```python
from build123d import *

# Parameters (mm, degrees)
BOSS_EXTRUDE1_DEPTH        = 19.05
BOSS_EXTRUDE2_DEPTH        = 19.05
FILLET1_R                  = 3.175
FILLET2_R                  = 12.7
CUT_EXTRUDE1_DEPTH         = 965.552600368
CUT_EXTRUDE1_DEPTH_BACK    = 965.552600368
SKETCH47_R                 = 3.175
FILLET4_R                  = 6.35
F_0_25_DIAMETER_HOLE1_D    = 6.35
HOLE6_D                    = 3.175
HOLE6_DEPTH                = 38.1
HOLE6_CSINK_D              = 10.16
HOLE6_CSINK_ANGLE          = 82
HOLE6_TIP                  = 0.953866233
HOLE9_D                    = 3.175
HOLE9_DEPTH                = 57.15
HOLE9_CSINK_D              = 10.16
HOLE9_CSINK_ANGLE          = 82
HOLE9_TIP                  = 0.953866233
HOLE14_D                   = 3.175
HOLE14_DEPTH               = 31.75
HOLE14_CSINK_D             = 10.16
HOLE14_CSINK_ANGLE         = 82
HOLE14_TIP                 = 0.953866233
HOLE15_D                   = 3.175
HOLE15_DEPTH               = 31.75
HOLE15_CSINK_D             = 10.16
HOLE15_CSINK_ANGLE         = 82
HOLE15_TIP                 = 0.953866233
HOLE17_D                   = 3.175
HOLE17_DEPTH               = 31.75
HOLE17_CSINK_D             = 10.16
HOLE17_CSINK_ANGLE         = 82
HOLE17_TIP                 = 0.953866233
F_1_2_0_5_DIAMETER_HOLE3_D = 12.7


with BuildPart() as part:
    # Sketch1 → Boss-Extrude1 (new body)
    with BuildSketch(Plane.XY):
        Polygon((-247.274665566, 82.142339986), (-327.22102196, 55.917162383), (-560.337153612, 766.561933763), (-504.525442447, 784.870110692), (-417.251419261, 518.818903446), (-393.116774032, 526.735904121), align=None)
    extrude(amount=-BOSS_EXTRUDE1_DEPTH)

    # Sketch2 → Boss-Extrude2 (add, through all)
    with BuildSketch(Plane.XY):
        Polygon((-393.116774032, 526.735904121), (-336.901176267, 355.36500697), (-277.604402796, 374.816405204), (-281.415155825, 417.005352091), (-320.44916939, 493.083731154), (-290.280862854, 502.979981998), (-307.307307279, 554.884385267), align=None)
    extrude(amount=-BOSS_EXTRUDE2_DEPTH)

    # Fillet1
    fillet1_edges = [part.edges().sort_by_distance(p)[0] for p in [
        (-320.44916939, 493.083731154, -9.525),
    ]]
    fillet(fillet1_edges, radius=FILLET1_R)

    # Fillet2
    fillet2_edges = [part.edges().sort_by_distance(p)[0] for p in [
        (-336.901176267, 355.36500697, -9.525),
    ]]
    fillet(fillet2_edges, radius=FILLET2_R)

    # Sketch47 → Cut-Extrude1 (cut, two sides: drawn at the far end of the back side and taken through both)
    with BuildSketch(Plane(origin=(0, 0, -19.05), x_dir=(-1, 0, 0), z_dir=(0, 0, -1)).offset(-CUT_EXTRUDE1_DEPTH_BACK)):
        with Locations((417.251419261, 518.818903446)):
            Circle(SKETCH47_R)
    extrude(amount=CUT_EXTRUDE1_DEPTH + CUT_EXTRUDE1_DEPTH_BACK, mode=Mode.SUBTRACT)

    # Fillet4
    fillet4_edges = [part.edges().sort_by_distance(p)[0] for p in [
        (-418.241044345, 521.8357341, -9.525),
        (-414.234588607, 519.80852853, -9.525),
    ]]
    fillet(fillet4_edges, radius=FILLET4_R)

    # 0.25_ Diameter Hole1 (through all)
    with Locations(Plane.XY):
        with Locations((-563.45033927, 698.544682362), (-504.072834209, 517.534843147), (-343.557230523, 532.968767209), (-316.40575464, 541.875392969), (-305.317060721, 508.071973621), (-332.468536604, 499.165347862), (-384.427899865, 457.805801818), (-325.157897499, 477.248418201), (-305.715281117, 417.978415836), (-364.985283482, 398.535799453), (-323.698740376, 393.110483865), (-289.824308357, 404.222472403), (-287.772364418, 381.505347156), (-316.771364786, 371.99266929)):
            Hole(F_0_25_DIAMETER_HOLE1_D / 2)

    # Hole6
    with Locations(Plane(origin=(313.774034822, -375.700785937, -19.05), x_dir=(-0.9977564584489054, 0.06694811142592419, 0), z_dir=(0, 0, -1))):
        with Locations((615.24080496, 429.781381762), (710.914924699, 391.126528253), (904.68821492, 1078.38439498), (976.811864753, 1049.244548945), (835.937309391, 717.51890547), (711.83598555, 767.659094962)):
            CounterSinkHole(HOLE6_D / 2, HOLE6_CSINK_D / 2, depth=HOLE6_DEPTH, counter_sink_angle=HOLE6_CSINK_ANGLE)
            with Locations((0, 0, -(HOLE6_DEPTH + HOLE6_TIP / 2))):  # 118° drill point
                Cone(0, HOLE6_D / 2, HOLE6_TIP, mode=Mode.SUBTRACT)

    # Hole9
    with Locations(Plane(origin=(313.774034822, -375.700785937, -38.1), x_dir=(-0.9977564584489054, 0.06694811142592419, 0), z_dir=(0, 0, -1))):
        with Locations((848.944412528, 940.413642522), (885.927448463, 1031.949868564), (867.435930496, 986.181755543), (830.452894561, 894.645529501)):
            CounterSinkHole(HOLE9_D / 2, HOLE9_CSINK_D / 2, depth=HOLE9_DEPTH, counter_sink_angle=HOLE9_CSINK_ANGLE)
            with Locations((0, 0, -(HOLE9_DEPTH + HOLE9_TIP / 2))):  # 118° drill point
                Cone(0, HOLE9_D / 2, HOLE9_TIP, mode=Mode.SUBTRACT)

    # Hole14
    with Locations(Plane(origin=(-45.102820315, -493.424841018, 72.024999997), x_dir=(0, 0, -1), z_dir=(0.9501828830204607, 0.31169293995040287, 1.2726359102629282e-15))):
        with Locations((174.999999994, 685.961004241), (174.999999994, 549.837259632), (174.999999994, 413.713515022), (81.549999997, 779.649723129), (81.549999997, 652.344645962), (62.499999997, 662.953402392), (62.499999997, 769.040966698), (-62.499999997, 769.040966698), (-62.499999997, 662.953402392), (-81.549999997, 652.344645962), (-81.549999997, 779.649723129), (-174.999999994, 413.713515022), (-174.999999994, 549.837259632), (-174.999999994, 685.961004241), (-82.737499997, 600.384620239), (0, 600.384620239), (82.737499997, 600.384620239), (0, 376.737770337), (-82.737499997, 376.737770337), (82.737499997, 376.737770337)):
            CounterSinkHole(HOLE14_D / 2, HOLE14_CSINK_D / 2, depth=HOLE14_DEPTH, counter_sink_angle=HOLE14_CSINK_ANGLE)
            with Locations((0, 0, -(HOLE14_DEPTH + HOLE14_TIP / 2))):  # 118° drill point
                Cone(0, HOLE14_D / 2, HOLE14_TIP, mode=Mode.SUBTRACT)

    # Hole15
    with Locations(Plane(origin=(-155.217483245, -529.546269464, 72.024999997), x_dir=(0, 0, 1), z_dir=(-0.9501828830204603, -0.3116929399504042, -1.2203303954814629e-15))):
        with Locations((-78.374999997, 1310.187770338), (-78.374999997, 1138.737770338), (78.374999997, 1138.737770338), (78.374999997, 1310.187770338)):
            CounterSinkHole(HOLE15_D / 2, HOLE15_CSINK_D / 2, depth=HOLE15_DEPTH, counter_sink_angle=HOLE15_CSINK_ANGLE)
            with Locations((0, 0, -(HOLE15_DEPTH + HOLE15_TIP / 2))):  # 118° drill point
                Cone(0, HOLE15_D / 2, HOLE15_TIP, mode=Mode.SUBTRACT)

    # Hole17
    with Locations(Plane(origin=(-111.425869636, 920.503328092, 72.024999997), x_dir=(0, 0, -1), z_dir=(-0.31169293995040415, 0.9501828830204603, 0))):
        with Locations((81.549999997, 448.336332751), (-81.549999997, 448.336332751)):
            CounterSinkHole(HOLE17_D / 2, HOLE17_CSINK_D / 2, depth=HOLE17_DEPTH, counter_sink_angle=HOLE17_CSINK_ANGLE)
            with Locations((0, 0, -(HOLE17_DEPTH + HOLE17_TIP / 2))):  # 118° drill point
                Cone(0, HOLE17_D / 2, HOLE17_TIP, mode=Mode.SUBTRACT)

    # 1/2 (0.5) Diameter Hole3 (through all)
    with Locations(Plane.XY):
        with Locations((-468.912808487, 528.603872083), (-528.290313547, 709.613711299)):
            Hole(F_1_2_0_5_DIAMETER_HOLE3_D / 2)


solid = part.part
```
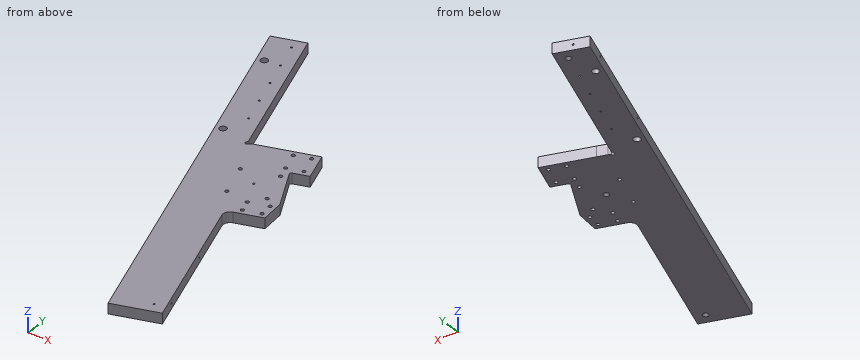
Build history of the part. All positions in model axes, mm. Round coordinates to 2 decimals unless told otherwise and drop trailing zeros. Write each loop counter-clockwise with the first axis right and the second up, starting at its lowest first coordinate (ties: lowest second). Pieces come first, ordered by that corner, then holes.
1) Pin check, flat tips, straight feed: pin 1 (4 mm diameter, centred on x = -364.99, y = 398.54, fed in from -Z); pin 2 (10 mm diameter, centred on y = 242, z = -13.5, fed in from +X); pin 3 (1.5 mm diameter, centred on y = 597, z = -2.5, fed in from -X); pin 4 (10 mm diameter, centred on y = 405.5, z = -9, fed in from +X). Stop position of each tip, or through.
2) Band-saw the part on B-B, the plane y = 199. List the corners of the cut face in (x, z).
3) Band-saw the part on A-A, the plane x = -438. List the corners of the cut face in (y, z).
4) Drill centre lines: probe 1 along X at (y, z) = (381, -9.75); probe 2 along X at (y, z) = (195, -5); probe 3 along X at (y, z) = (280.5, -16.75). Where is each one in solid material? Low to high.
Ans:
1. pin 1: passes through
1. pin 2: stops at x = -298.07
1. pin 3: stops at x = -504.96
1. pin 4: stops at x = -279.92
2. outline: (-374.16, -19.05) - (-285.61, -19.05) - (-285.61, 0) - (-374.16, 0) - close
3. outline: (393.62, -19.05) - (582.07, -19.05) - (582.07, 0) - (393.62, 0) - close
4. probe 1: x = -433.86 to -290.91, -284.64 to -278.16
4. probe 2: x = -372.85 to -284.3
4. probe 3: x = -400.89 to -312.34
